Input: part model. Units: mm. Frame: model coordinates. A direction names the side the tool comes from. Coordinates: 2 decimals unless noted, no trailing zeros. Loops run counter-clockwise (first coordinate to the right, second up) from the corner with the lowest first, then second, coordinate; pieces in that order, holes last. Notation, with made-up numbers: (25.25, -3.5) - (42.25, -3.5) arc R20 ccw to (42.25, 27.5) - close; hole circle Ø6 at (33.5, -18). An arc over 180 degrees is marked (long way). Use a Markdown table: item, result. Add a question column.
1. Section query D-D on z = 73. Return the cut outline in (x, y).
2. Section query A-A on y = 0. Return the cut outline in (x, z), then the cut area to 3 significant figures.
3. Section query C-C on z = 21. Return the cut outline in (x, y), then the cut area to 3 significant figures.
4. Ray query, L1, parallel to X at y = 5.5, z = 59; L2, parallel to Y at x = 6.5, z = 32.5; L3, parallel to Y at x = -9.25, z = 22. Return the intervals inside material, ascending. Write a range as [from, to].
5. Access query for faces 1 (the face through (-5.581, 5.653, 28.466)), 2 (the face through (-6.244, 6.344, 20.061)), 3 (the face through (9, 2.54, 43)), 4 (the face through (2.54, -9, 43)), 5 (the face through (5, -5, 37.139)). Directions: +Z, -Z, +X, -X, +Y, -Y. A direction counts if a zero-diameter tool reaches every point of the face in a straight line with its end or side. Return the directions, or none.
6. Contact query for flat-ended pins moving along their axis: P1, Ø3, axis at x = -7.5, z = 31.5, coming from the -Y side; P2, Ø1, axis at y = 4.5, z = 49.5, coming from the +X side; P3, Ø2.5, axis at x = 5.5, y = -6, coming from the -Z side. Output: stop coordinate, or through.
7. Draft query along X for faces 6 (the face through (-10, 0, 71.391)), 7 (the face through (6.344, 6.244, 20.061)). Return one class per face: released by +X, released by -X, zero draft, split by the parting line, or undercut.
```python
from build123d import *

# Parameters (mm, degrees)
CUT_EXTRUDE1_DEPTH      = 86.717666245
CUT_EXTRUDE1_DEPTH_BACK = 86.717666245
SKETCH7_W               = 5.08
SKETCH7_H               = 55.892291628
CUT_EXTRUDE2_DEPTH      = 86.717666245
CUT_EXTRUDE2_DEPTH_BACK = 86.717666245
SKETCH8_W               = 5.08
SKETCH8_H               = 55.892291628


with BuildPart() as part:
    # Sketch4 → Revolve1 (revolve)
    with BuildSketch(Plane.YZ, mode=Mode.PRIVATE) as revolve1_sk:
        Polygon((11.75385, 15.498209184), (11.75385, 84.090500812), (7.94385, 84.090500812), (7.94385, 37.139237028), (3.258679023, 37.139237028), (3.258679023, 32.283867455), (7.94385, 32.283867455), (7.94385, 24.752767455), (5.969, 24.752767455), align=None)
    revolve(revolve1_sk.sketch.rotate(Axis((0, 0, -23.885554531), (0, 0, 1)), 90), axis=Axis((0, 0, -23.885554531), (0, 0, 1)))

    # Sketch7 → Cut-Extrude1 (cut, two sides: drawn at the far end of the back side and taken through both)
    with BuildSketch(Plane.YZ.offset(-CUT_EXTRUDE1_DEPTH_BACK)):
        with Locations((0, 43.444354998)):
            Rectangle(SKETCH7_W, SKETCH7_H)
    extrude(amount=CUT_EXTRUDE1_DEPTH + CUT_EXTRUDE1_DEPTH_BACK, mode=Mode.SUBTRACT)

    # Sketch8 → Cut-Extrude2 (cut, two sides: drawn at the far end of the back side and taken through both)
    with BuildSketch(Plane(origin=(0, 0, 0), x_dir=(-1, 0, 0), z_dir=(0, 1, 0)).offset(-CUT_EXTRUDE2_DEPTH_BACK)):
        with Locations((0, 43.444354998)):
            Rectangle(SKETCH8_W, SKETCH8_H)
    extrude(amount=CUT_EXTRUDE2_DEPTH + CUT_EXTRUDE2_DEPTH_BACK, mode=Mode.SUBTRACT)


solid = part.part
```
Resolved:
| question | item | result |
|---|---|---|
| 1 | outline | circle Ø23.51 at (0, 0); hole circle Ø15.89 at (0, 0) |
| 2 | outline | (-11.75, 71.39) - (-7.94, 71.39) - (-7.94, 84.09) - (-11.75, 84.09) - close; (7.94, 71.39) - (11.75, 71.39) - (11.75, 84.09) - (7.94, 84.09) - close |
| 2 | area | 96.8 mm² |
| 3 | outline | (-11.48, -2.54) arc R11.75 ccw to (-2.54, -11.48) - (-2.54, -7.92) arc R8.31 cw to (-7.92, -2.54) - close; (-11.48, 2.54) - (-7.92, 2.54) arc R8.31 cw to (-2.54, 7.92) - (-2.54, 11.48) arc R11.75 ccw to start; (2.54, -11.48) arc R11.75 ccw to (11.48, -2.54) - (7.92, -2.54) arc R8.31 cw to (2.54, -7.92) - close; (2.54, 7.92) arc R8.31 cw to (7.92, 2.54) - (11.48, 2.54) arc R11.75 ccw to (2.54, 11.48) - close |
| 3 | area | 146 mm² |
| 4 | L1 | [-10.39, -5.73], [5.73, 10.39] |
| 4 | L2 | [-9.79, -2.54], [2.54, 9.79] |
| 4 | L3 | [-7.25, -2.54], [2.54, 7.25] |
| 5 | face 1 | none |
| 5 | face 2 | -Z |
| 5 | face 3 | -Z, +X, -X |
| 5 | face 4 | -Z, +Y, -Y |
| 5 | face 5 | +Z |
| 6 | P1 | y = -10.11 |
| 6 | P2 | x = 11.05 |
| 6 | P3 | z = 19.28 |
| 7 | face 6 | zero draft |
| 7 | face 7 | undercut |
